Geometry: see drawing. Coordinates: mm, zero at the bounding-box minimum. Give positions to 0.01 mm unless a question says otherwise; leave off trailing zeros. Order: outer loops, then holes, each group sorted by start corner. A loop starts at its lowest first (then second) coordinate and runs counter-clockwise, first axis right, second up. Notation, with made-up numbers: (-11.5, -20) - (24.5, -20) arc R6 cw to (24.5, -11) - close; hole circle Ø9 at (24.25, -6). An arc over 180 degrees is marked (long way). Write item = value, one per line. Start each with the question number.
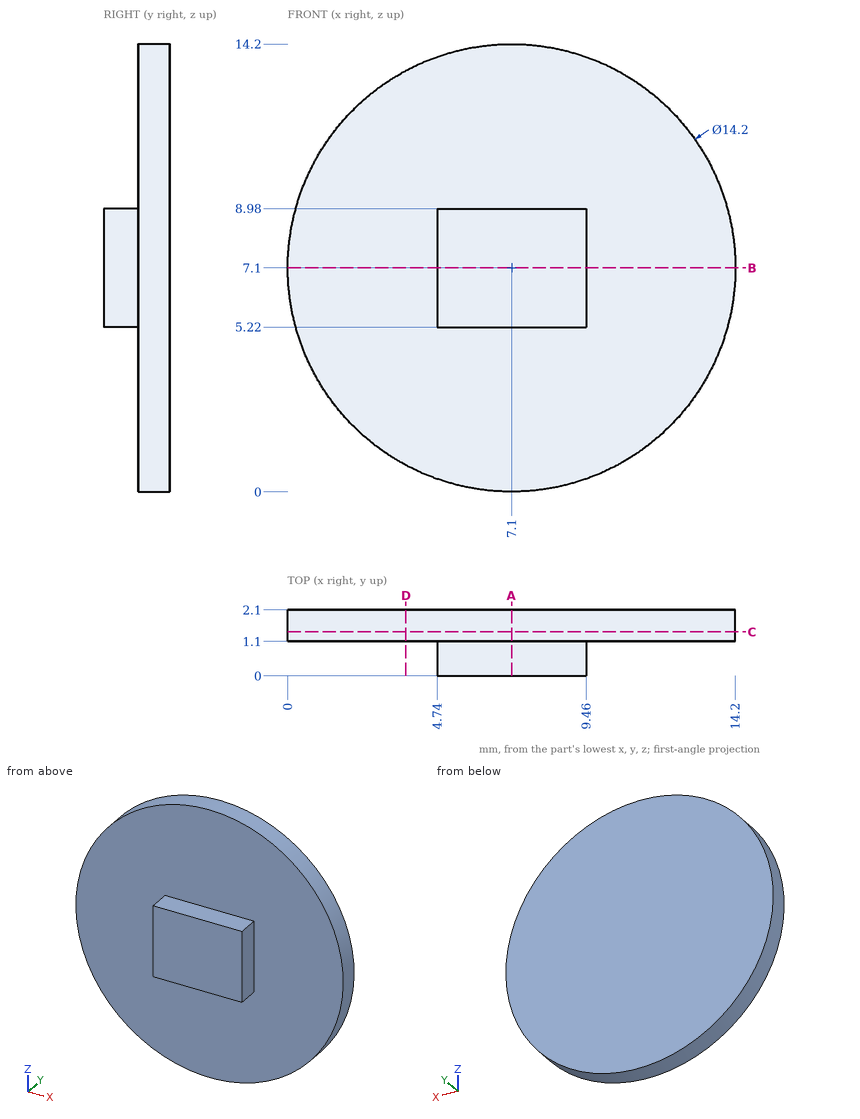
Q1. Section C-C, the plane y = 1.4. Return the cut outline in (x, z), then the cut area to 3 significant figures.
Q2. Section B-B, the plane z = 7.1. Return the cut outline in (x, y).
Q3. Section D-D, the plane x = 3.75. Return the cut outline in (y, z).
Q4. Material intervals for line 1 along Y through (x, z) = (9.25, 3.5); line 2 along Z through (x, y) = (5.25, 0.6); line 3 along X through (y, z) = (0.3, 8.75), sorted ascending. Write a range as from..to.
Q5. Contact query for flat-ended pins moving along their axis: pin 1 (0.9 mm diameter, centred on y = 0.5, z = 7, fed in from +X); pin 2 (4.5 mm diameter, centred on x = 7, z = 10.5, fed in from -Y); pin 3 (6 mm diameter, centred on x = 5.5, z = 2, fed in from -Y). Output: stop coordinate, or through.
Q6. Section A-A, the plane x = 7.1. Return the cut outline in (y, z).
The answers:
q1.outline = circle Ø14.2 at (7.1, 7.1)
q1.area = 158 mm²
q2.outline = (0, 1.1) - (4.74, 1.1) - (4.74, 0) - (9.46, 0) - (9.46, 1.1) - (14.2, 1.1) - (14.2, 2.1) - (0, 2.1) - close
q3.outline = (1.1, 0.84) - (2.1, 0.84) - (2.1, 13.36) - (1.1, 13.36) - close
q4.line_1 = 1.1..2.1
q4.line_2 = 5.22..8.98
q4.line_3 = 4.74..9.46
q5.pin_1 = 9.46
q5.pin_2 = 0
q5.pin_3 = 1.1
q6.outline = (0, 5.22) - (1.1, 5.22) - (1.1, 0) - (2.1, 0) - (2.1, 14.2) - (1.1, 14.2) - (1.1, 8.98) - (0, 8.98) - close
